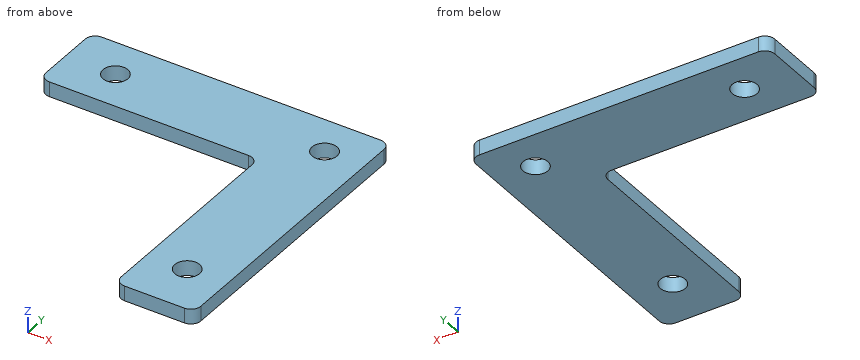
```python
from build123d import *

# Parameters (mm, degrees)
BOSS_EXTRUDE1_DEPTH   = 3
SKETCH2_R             = 2.5
CUT_EXTRUDE1_DEPTH    = 3
FILLET1_R             = 2
F_5_0MM_DOWEL_HOLE1_D = 5


with BuildPart() as part:
    # Sketch1 → Boss-Extrude1 (new body)
    with BuildSketch(Plane.XY):
        Polygon((0, 0), (44, 0), (44, -44), (60, -44), (60, -15.656804173), (60, 16), (0, 16), align=None)
    extrude(amount=BOSS_EXTRUDE1_DEPTH)

    # Sketch2 → Cut-Extrude1 (cut)
    with BuildSketch(Plane.XY.offset(3)):
        with Locations((10, 8)):
            Circle(SKETCH2_R)
        with Locations((52, -34)):
            Circle(SKETCH2_R)
    extrude(amount=-CUT_EXTRUDE1_DEPTH, mode=Mode.SUBTRACT)

    # Fillet1
    fillet1_edges = [part.edges().sort_by_distance(p)[0] for p in [
        (0, 16, 1.5),
        (60, 16, 1.5),
        (60, -44, 1.5),
        (44, -44, 1.5),
        (44, 0, 1.5),
        (0, 0, 1.5),
    ]]
    fillet(fillet1_edges, radius=FILLET1_R)

    # Ø5.0mm Dowel Hole1 (through all)
    with Locations(Plane(origin=(0, 0, 0), x_dir=(-1, 0, 0), z_dir=(0, 0, -1))):
        with Locations((-52, 8)):
            Hole(F_5_0MM_DOWEL_HOLE1_D / 2)


solid = part.part
```
The listing builds one solid part. Answer for the finished solid, in the listing's coordinates (mm). Round coordinates to 2 decimals unless told otherwise and drop trailing zeros. Loops run counter-clockwise (first coordinate to the right, second up) from the corner with the lowest first, then second, coordinate; pieces in that order, holes last. Notation, with made-up numbers: (-21.75, 2.5) - (21.25, 2.5) arc R29 ccw to (21.25, 38.5) - close; hole circle Ø6 at (-16, 27). An arc over 180 degrees is marked (long way). Use one line per item in the form item = value. Start each with the question number.
1. Given pin 1 Ø4 at (x, y) = (52, -34) entering from -Z; pin 2 Ø1.5 at (x, z) = (17.5, 1) entering from -Y, each flat-ended and moving along its own axis, determine where each tip first touches the part or whether it passes through.
2. The part is cut by section A-A on x = 52. Determine the outline of the cut face in (y, z), then the cut area to 3 significant figures.
3. The part is cut by section B-B on y = 8. Determine the outline of the cut face in (x, z).
4. The part is cut by section D-D on x = 10. Determine the outline of the cut face in (y, z), then the cut area to 3 significant figures.
5. The part is cut by section C-C on z = 2.45. Determine the outline of the cut face in (x, y), then the cut area to 3 significant figures.
6. Consider line 1 (Y direction, x = 52, z = 1.4); line 2 (Y direction, x = 10, z = 1.25); line 3 (X direction, y = -4, z = 2.1). Determine where each line is inside the solid, lowest interval first. Write a range as [from, to].
Geometry check:
q1.pin_1 = through
q1.pin_2 = 0
q2.outline = (-44, 0) - (-36.5, 0) - (-36.5, 3) - (-44, 3) - close; (-31.5, 0) - (5.5, 0) - (5.5, 3) - (-31.5, 3) - close; (10.5, 0) - (16, 0) - (16, 3) - (10.5, 3) - close
q2.area = 150 mm^2
q3.outline = (0, 0) - (7.5, 0) - (7.5, 3) - (0, 3) - close; (12.5, 0) - (49.5, 0) - (49.5, 3) - (12.5, 3) - close; (54.5, 0) - (60, 0) - (60, 3) - (54.5, 3) - close
q4.outline = (0, 0) - (5.5, 0) - (5.5, 3) - (0, 3) - close; (10.5, 0) - (16, 0) - (16, 3) - (10.5, 3) - close
q4.area = 33.0 mm^2
q5.outline = (0, 2) arc R2 ccw to (2, 0) - (42, 0) arc R2 cw to (44, -2) - (44, -42) arc R2 ccw to (46, -44) - (58, -44) arc R2 ccw to (60, -42) - (60, 14) arc R2 ccw to (58, 16) - (2, 16) arc R2 ccw to (0, 14) - close; hole circle Ø5 at (10, 8); hole circle Ø5 at (52, -34); hole circle Ø5 at (52, 8)
q5.area = 1,600 mm^2
q6.line_1 = [-44, -36.5], [-31.5, 5.5], [10.5, 16]
q6.line_2 = [0, 5.5], [10.5, 16]
q6.line_3 = [44, 60]
